from build123d import *

# Parameters (mm, degrees)
ESQUISSE1_W      = 80
ESQUISSE1_H      = 80
ESQUISSE1_R      = 2.5
EXTRUSION1_DEPTH = 3
CONG_1_R         = 2


with BuildPart() as part:
    # Esquisse1 → Extrusion1 (new body)
    with BuildSketch(Plane(origin=(0, 0, 0), x_dir=(1, 0, 0), z_dir=(0, 1, 0))):
        with Locations((40, 40)):
            Rectangle(ESQUISSE1_W, ESQUISSE1_H)
        with Locations((40, 40)):
            Circle(ESQUISSE1_R, mode=Mode.SUBTRACT)
        with Locations((60, 40)):
            Circle(ESQUISSE1_R, mode=Mode.SUBTRACT)
    extrude(amount=EXTRUSION1_DEPTH)

    # Congé1
    cong_1_edges = [part.edges().sort_by_distance(p)[0] for p in [
        (0, 1.5, -80),
        (80, 1.5, -80),
        (80, 1.5, 0),
        (0, 1.5, 0),
    ]]
    fillet(cong_1_edges, radius=CONG_1_R)


solid = part.part
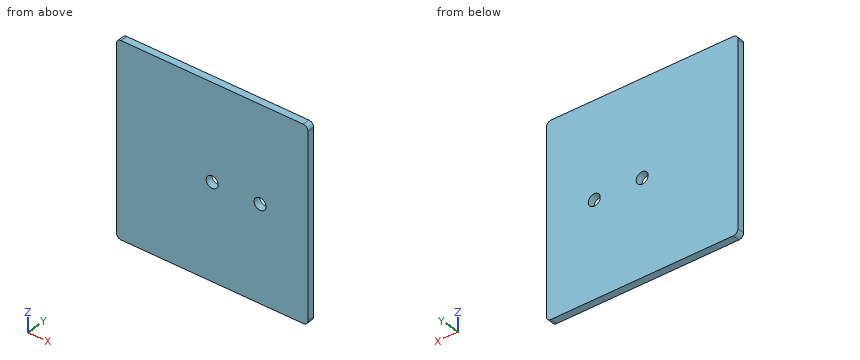
Build history of the part. All positions in model axes, mm. Round coordinates to 2 decimals unless told otherwise and drop trailing zeros. Write each loop counter-clockwise with the first axis right and the second up, starting at its lowest first coordinate (ties: lowest second). Pieces come first, ordered by that corner, then holes. Notation, with made-up numbers: (41.25, 67.25) -> (68.25, 67.25) arc R25 cw to (68.25, 82.25) -> close; hole circle Ø7 at (70.5, 64). An arc over 180 degrees is marked (long way). Write item = value, one per line.
(1) Band-saw the part on B-B (z = -40). Give the cut face in (x, y).
Answer:
outline = (0, 0) -> (37.5, 0) -> (37.5, 3) -> (0, 3) -> close; (42.5, 0) -> (57.5, 0) -> (57.5, 3) -> (42.5, 3) -> close; (62.5, 0) -> (80, 0) -> (80, 3) -> (62.5, 3) -> close
(2) Band-saw the part on A-A (x = 40). Give the cut face in (y, z), then the cut area to 3 significant figures.
Answer:
outline = (0, -80) -> (3, -80) -> (3, -42.5) -> (0, -42.5) -> close; (0, -37.5) -> (3, -37.5) -> (3, 0) -> (0, 0) -> close
area = 225 mm2
(3) Flat gauge pin, fed straight in: pin 1 (5 mm diameter, centred on x = 17.5, z = -14.5, fed in from -Y). Where does the tip first touch, or does it go through?
Answer:
pin_1 = 0
(4) Probe L1, parallel to X at y = 1.25, z = -40; L2, parallel to Z at x = 40, y = 0.85; L3, parallel to X at y = 0.9, z = -38. List the from-to ranges inside material, lowest first.
Answer:
L1 = 0 to 37.5, 42.5 to 57.5, 62.5 to 80
L2 = -80 to -42.5, -37.5 to 0
L3 = 0 to 38.5, 41.5 to 58.5, 61.5 to 80
